Read the model definition and answer for the solid it produces. Units are mm, in the model's axes. A direction names the side the tool comes from. Coordinates: 2 decimals unless noted, no trailing zeros. Order: outer loops, then holes, each group sorted by start corner. A loop starts at its lowest first (then second) coordinate and runs counter-clockwise, first axis right, second up.
```python
from build123d import *

# Parameters (mm, degrees)
SZKIC1_W                         = 20
SZKIC1_H                         = 8
DODANIE_WYCI_GNI_CIE1_DEPTH      = 350
SZKIC2_R                         = 12
DODANIE_WYCI_GNI_CIE2_DEPTH      = 5
DODANIE_WYCI_GNI_CIE3_START      = 5
SZKIC3_R                         = 12
DODANIE_WYCI_GNI_CIE3_DEPTH      = 5
DODANIE_WYCI_GNI_CIE4_DEPTH      = 8
DODANIE_WYCI_GNI_CIE4_DEPTH_BACK = 16
SZKIC6_R                         = 6
DODANIE_WYCI_GNI_CIE5_DEPTH      = 65
SZKIC7_R                         = 6
DODANIE_WYCI_GNI_CIE6_DEPTH      = 65
SZKIC8_R                         = 20
SZKIC8_R_2                       = 14
DODANIE_WYCI_GNI_CIE7_DEPTH      = 300
SZKIC13_R                        = 20
SZKIC13_R_2                      = 14
WYTNIJ_WYCI_GNI_CIE1_DEPTH       = 50
DODANIE_WYCI_GNI_CIE9_DEPTH      = 20
DODANIE_WYCI_GNI_CIE9_DEPTH_BACK = 20
WYTNIJ_WYCI_GNI_CIE2_DEPTH       = 40
SZKIC16_R                        = 6
DODANIE_WYCI_GNI_CIE10_DEPTH     = 40


with BuildPart() as part:
    # Szkic1 → Dodanie-wyci_gni_cie1 (new body)
    with BuildSketch(Plane.XY):
        Rectangle(SZKIC1_W, SZKIC1_H)
    extrude(amount=DODANIE_WYCI_GNI_CIE1_DEPTH)

    # Szkic2 → Dodanie-wyci_gni_cie2 (add)
    with BuildSketch(Plane.XY.offset(350)):
        Circle(SZKIC2_R)
    extrude(amount=DODANIE_WYCI_GNI_CIE2_DEPTH)

    # Szkic3 → Dodanie-wyci_gni_cie3 (add)
    with BuildSketch(Plane(origin=(0, 0, 0), x_dir=(-1, 0, 0), z_dir=(0, 0, -1)).offset(DODANIE_WYCI_GNI_CIE3_START)):
        with Locations(Location((0, 0, 0), (0, 0, 180))):
            Circle(SZKIC3_R)
    extrude(amount=-DODANIE_WYCI_GNI_CIE3_DEPTH)

    # Szkic5 → Dodanie-wyci_gni_cie4 (add, two sides: drawn at the far end of the back side and taken through both)
    with BuildSketch(Plane(origin=(0, 4, 0), x_dir=(1, 0, 0), z_dir=(0, 1, 0)).offset(-DODANIE_WYCI_GNI_CIE4_DEPTH_BACK)):
        Polygon((-12, -350), (12, -350), (12, -357.522501646), (-12, -355), align=None)
    extrude(amount=DODANIE_WYCI_GNI_CIE4_DEPTH + DODANIE_WYCI_GNI_CIE4_DEPTH_BACK)

    # Szkic6 → Dodanie-wyci_gni_cie5 (add)
    with BuildSketch(Plane(origin=(-37.035439516, 0, 352.368669275), x_dir=(0.9945218953682733, 0, 0.1045284632676537), z_dir=(-0.1045284632676537, 0, 0.9945218953682733))):
        with Locations(Location((37.23944107, 0, 0), (0, 0, 180))):
            Circle(SZKIC6_R)
    extrude(amount=DODANIE_WYCI_GNI_CIE5_DEPTH)

    # Szkic7 → Dodanie-wyci_gni_cie6 (add)
    with BuildSketch(Plane(origin=(0, 0, -5), x_dir=(-1, 0, 0), z_dir=(0, 0, -1))):
        Circle(SZKIC7_R)
    extrude(amount=DODANIE_WYCI_GNI_CIE6_DEPTH)

    # Szkic8 → Dodanie-wyci_gni_cie7 (add)
    with BuildSketch(Plane(origin=(0, 0, 350), x_dir=(-1, 0, 0), z_dir=(0, 0, -1))):
        Circle(SZKIC8_R)
        with Locations(Location((0, 0, 0), (0, 0, 148.997280866))):
            Circle(SZKIC8_R_2, mode=Mode.SUBTRACT)
    extrude(amount=DODANIE_WYCI_GNI_CIE7_DEPTH)

    # Szkic13 → Wytnij-wyci_gni_cie1 (cut)
    with BuildSketch(Plane.XY.offset(350)):
        Circle(SZKIC13_R)
        Circle(SZKIC13_R_2, mode=Mode.SUBTRACT)
    extrude(amount=-WYTNIJ_WYCI_GNI_CIE1_DEPTH, mode=Mode.SUBTRACT)


with BuildPart() as wytnij_wyci_gni_cie1_piece_1:
    # of the separate pieces the step leaves, piece 1, a body of its own (wytnij_wyci_gni_cie1_pieces)
    add(part.part.solids().sort_by_distance((12, 7.211102551, 300))[0])



with BuildPart() as wytnij_wyci_gni_cie1_piece_2:
    # of the separate pieces the step leaves, piece 2, a body of its own (wytnij_wyci_gni_cie1_pieces)
    add(part.part.solids().sort_by_distance((12, 0, -5))[0])


with BuildPart() as wytnij_wyci_gni_cie1_piece_1_1:
    add(wytnij_wyci_gni_cie1_piece_1.part)

    add(wytnij_wyci_gni_cie1_piece_2.part)  # Dodanie-wyci_gni_cie9 merges Wytnij-wyci_gni_cie1 piece 2
    # Szkic14 → Dodanie-wyci_gni_cie9 (add, two sides: drawn at the far end of the back side and taken through both)
    with BuildSketch(Plane(origin=(0, 0, 0), x_dir=(0, 0, -1), z_dir=(1, 0, 0)).offset(-DODANIE_WYCI_GNI_CIE9_DEPTH_BACK)):
        Polygon((-175, 35), (-160, 35), (-160, 0), (-190, 0), (-190, 35), align=None)
    extrude(amount=DODANIE_WYCI_GNI_CIE9_DEPTH + DODANIE_WYCI_GNI_CIE9_DEPTH_BACK)

    # Szkic15 → Wytnij-wyci_gni_cie2 (cut)
    with BuildSketch(Plane(origin=(20, 0, 0), x_dir=(0, 0, -1), z_dir=(1, 0, 0))):
        with BuildLine():
            Line((-190, 35), (-190, 20))
            ThreePointArc((-190, 20), (-185.606601718, 30.606601718), (-175, 35))
            Line((-175, 35), (-190, 35))
        make_face()
        with BuildLine():
            ThreePointArc((-175, 35), (-164.393398282, 30.606601718), (-160, 20))
            Line((-160, 20), (-160, 35))
            Line((-160, 35), (-175, 35))
        make_face()
    extrude(amount=-WYTNIJ_WYCI_GNI_CIE2_DEPTH, mode=Mode.SUBTRACT)

    # Szkic16 → Dodanie-wyci_gni_cie10 (add)
    with BuildSketch(Plane(origin=(20, 0, 0), x_dir=(0, 0, -1), z_dir=(1, 0, 0))):
        with Locations(Location((-175, 20, 0), (0, 0, 180))):
            Circle(SZKIC16_R)
    extrude(amount=DODANIE_WYCI_GNI_CIE10_DEPTH)


solid = wytnij_wyci_gni_cie1_piece_1_1.part
```
1) A cutting plane is placed at C-C, the plane z = -24.5. Determine the outline of the cut face in (x, y).
A:
outline: circle Ø12 at (0, 0)
2) Straight lines are drawn through the part: line 1 (Y direction, x = 0, z = 202.5); line 2 (X direction, y = 0, z = 133); line 3 (Y direction, x = -8, z = 42). For each, find the intervals that lie inside material, in ascending order.
A:
line 1: y = -20 to -14, -4 to 4, 14 to 20
line 2: x = -20 to -14, -10 to 10, 14 to 20
line 3: y = -4 to 4
3) A cutting plane is placed at A-A, the plane z = 283.5. Determine the outline of the cut face in (x, y), and give its area (3 significant figures).
A:
outline: circle Ø40 at (0, 0); (-10, -4) - (10, -4) - (10, 4) - (-10, 4) - close; hole circle Ø28 at (0, 0)
area: 801 mm2
4) Which of the six approach directions +Z, -Z, +X, -X, +Y, -Y give full straight-line access (tool end or side, diameter ignored) to faces 1 (the cylindrical face through (6, 0, -37)), 2 (the flat face through (-15, 16, 160)), 3 (the cylindrical face through (5.588, -12.837, 176.75)), 4 (the flat face through (12, 0, 354)), 5 (the flat face through (16, 16, 190))?
A:
face 1: -Z
face 2: -Z, -X, +Y
face 3: none
face 4: +Z, +X, +Y, -Y
face 5: +Z, +X, +Y
5) Flat-ended cylindrical pins translate along their axes: pin 1 Ø10 at (x, y) = (-5.5, 10) entering from -Z; pin 2 Ø4 at (y, z) = (-1, 353) entering from +X; pin 3 Ø3 at (x, z) = (6, -15) entering from +Y. Find the tip coordinate at first contact, or state that the pin passes through.
A:
pin 1: stops at z = -5
pin 2: stops at x = 12
pin 3: stops at y = 3.97
6) A cutting plane is placed at B-B, the plane x = 24.5. Determine the outline of the cut face in (y, z), and give its area (3 significant figures).
A:
outline: circle Ø12 at (20, 175)
area: 113 mm2
7) Determine the mould class of faces 6 (the flat face through (-6.711, -0.084, 420.914)), 7 (the cylindrical face through (4.336, -19.524, 176.75)), 8 (the flat face through (0, 7, 160)) for opening direction X: pulls with the +X half, pulls with the -X half, needs draft (parallel to the pull), parting line crosses it, or undercut.
A:
face 6: pulls with the -X half
face 7: parting line crosses it
face 8: undercut
